Check sheet for the drawn part. Datum: minimum x, y, z corner. Units: mm. A direction names the side the tool comes from. Give positions to 0.01 mm unless a question says otherwise; leave off trailing zeros. Write each loop counter-clockwise with the first axis right and the second up, starting at its lowest first coordinate (ties: lowest second). Pieces come first, ordered by that corner, then holes.
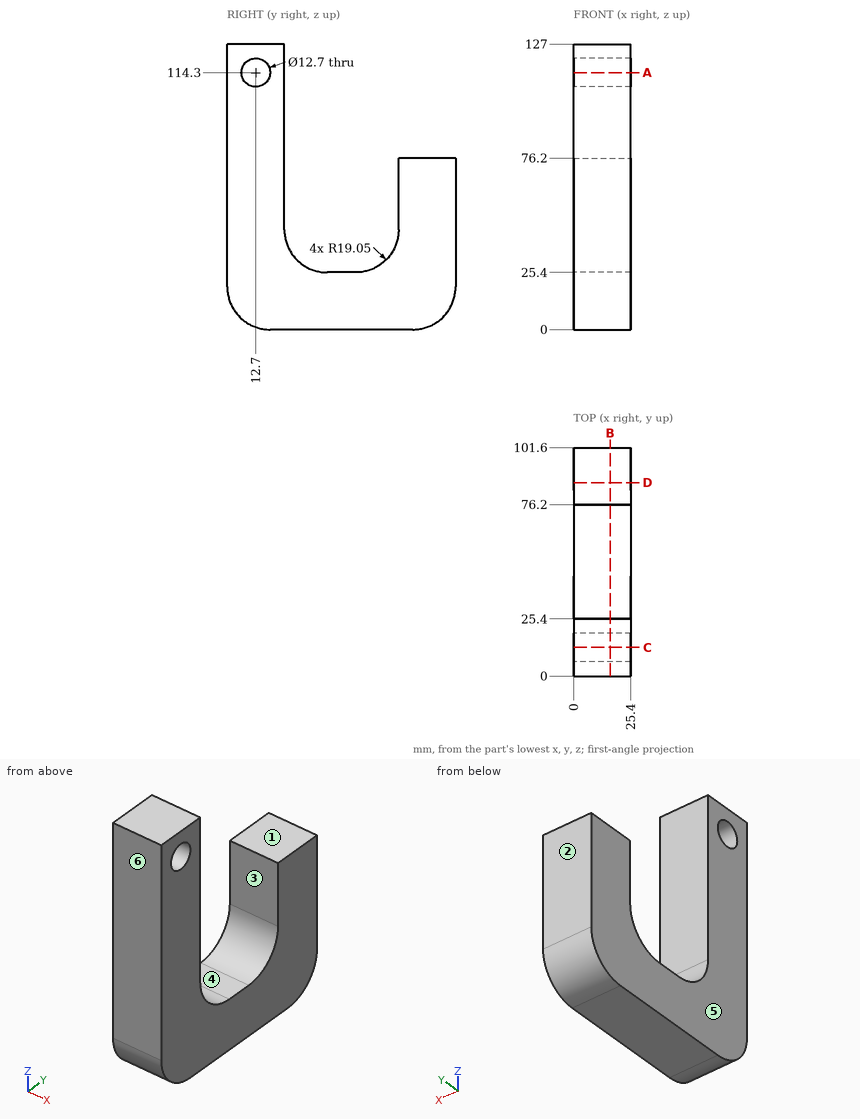
1) Sectioned sample at A-A on z = 114.3. Record the boundary of the cut face in (x, y).
2) Gauge pin test, flat ends, axial feed: pin 1 (6 mm diameter, centred on x = 7.5, y = 77.5, fed in from +Z); pin 2 (14 mm diameter, centred on x = 16, y = 48, fed in from +Z) (3 decimals); pin 3 (10 mm diameter, centred on x = 17.5, y = 56, fed in from -Z). Record the tip position at first contact, or that the pin passes through.
3) Draft check along Y on the marked faces 4, 5 and 6. Enter one of: +Y half, -Y half, draft (parallel to the pull), parting line (faces both ways), or undercut.
4) Sectioned sample at C-C on y = 12.7. Record the boundary of the cut face in (x, z).
5) Sectioned sample at B-B on x = 16.25. Record the boundary of the cut face in (y, z), then the cut area to 3 significant figures.
6) Scan lines: L1, parallel to Y at x = 15.75, z = 50; L2, parallel to Z at x = 10, y = 12.7; L3, parallel to Z at x = 21.75, y = 78.5. Record each from-to range of solid material in increasing order.
7) Access from +Z, -Z, +X, -X, +Y, -Y to the whole of each face (thin tool, end or side, straight path). Record for the marked faces 1, 2 and 3.
8) Sectioned sample at D-D on y = 86. Record the boundary of the cut face in (x, z) (3 decimals).
Answers below:
1. outline: (0, 0) - (25.4, 0) - (25.4, 6.35) - (0, 6.35) - close; (0, 19.05) - (25.4, 19.05) - (25.4, 25.4) - (0, 25.4) - close
2. pin 1: stops at z = 76.2
2. pin 2: stops at z = 25.715
2. pin 3: stops at z = 0
3. face 4: undercut
3. face 5: draft
3. face 6: -Y half
4. outline: (0, 1.09) - (25.4, 1.09) - (25.4, 107.95) - (0, 107.95) - close; (0, 120.65) - (25.4, 120.65) - (25.4, 127) - (0, 127) - close
5. outline: (0, 19.05) arc R19.05 ccw to (19.05, 0) - (82.55, 0) arc R19.05 ccw to (101.6, 19.05) - (101.6, 76.2) - (76.2, 76.2) - (76.2, 44.45) arc R19.05 cw to (57.15, 25.4) - (44.45, 25.4) arc R19.05 cw to (25.4, 44.45) - (25.4, 127) - (0, 127) - close; hole circle Ø12.7 at (12.7, 114.3)
5. area: 6,320 mm2
6. L1: y = 0 to 25.4, 76.2 to 101.6
6. L2: z = 1.09 to 107.95, 120.65 to 127
6. L3: z = 0 to 76.2
7. face 1: +Z, +X, -X, +Y
7. face 2: +Z, -Z, +X, -X, +Y
7. face 3: +Z, +X, -X
8. outline: (0, 0.315) - (25.4, 0.315) - (25.4, 76.2) - (0, 76.2) - close
